Can you work these out from the model? Positions are in its coordinate system, mm. Give positions to 0.01 mm unless a question says otherwise; leave off trailing zeros. Write each loop counter-clockwise with the first axis right and the second up, starting at its lowest first coordinate (ties: lowest second). Pieces come first, ordered by that corner, then holes.
1. Suppose I cut it at B-B (z = -0.4). Please give me the cut outline in (x, y), and give its area (3 significant figures).
2. Suppose I cut it at A-A (x = -38.1). Please give me the cut outline in (y, z).
3. Suppose I cut it at D-D (x = 12.7). Please give me the cut outline in (y, z), and give its area (3 significant figures).
4. Suppose I cut it at C-C (y = 12.7). Please give me the cut outline in (x, z).
5. If I drill on probe 1 along X at (y, z) = (12.7, 1.25); probe 2 along X at (y, z) = (13, 0.7); probe 3 along Y at (x, z) = (12.7, 0.85), over which ranges is the centre line in solid material (lowest first)?
```python
from build123d import *

# Parameters (mm, degrees)
SKETCH1_R           = 3.2639
BOSS_EXTRUDE1_DEPTH = 2.38125


with BuildPart() as part:
    # Sketch1 → Boss-Extrude1 (new, symmetric)
    with BuildSketch(Plane.XY):
        Polygon((76.2, 25.4), (25.4, 76.2), (0, 76.2), (-50.8, 25.4), (-50.8, 0), (0, 0), (76.2, 0), align=None)
        with Locations(Location((12.7, 12.7, 0), (0, 0, 180))):
            Circle(SKETCH1_R, mode=Mode.SUBTRACT)
        with Locations(Location((38.1, 12.7, 0), (0, 0, 180))):
            Circle(SKETCH1_R, mode=Mode.SUBTRACT)
        with Locations(Location((63.5, 12.7, 0), (0, 0, 180))):
            Circle(SKETCH1_R, mode=Mode.SUBTRACT)
        with Locations(Location((12.7, 38.1, 0), (0, 0, 180))):
            Circle(SKETCH1_R, mode=Mode.SUBTRACT)
        with Locations(Location((12.7, 63.5, 0), (0, 0, 180))):
            Circle(SKETCH1_R, mode=Mode.SUBTRACT)
        with Locations(Location((-38.1, 12.7, 0), (0, 0, 180))):
            Circle(SKETCH1_R, mode=Mode.SUBTRACT)
        with Locations(Location((-12.7, 12.7, 0), (0, 0, 180))):
            Circle(SKETCH1_R, mode=Mode.SUBTRACT)
    extrude(amount=BOSS_EXTRUDE1_DEPTH, both=True)


solid = part.part
```
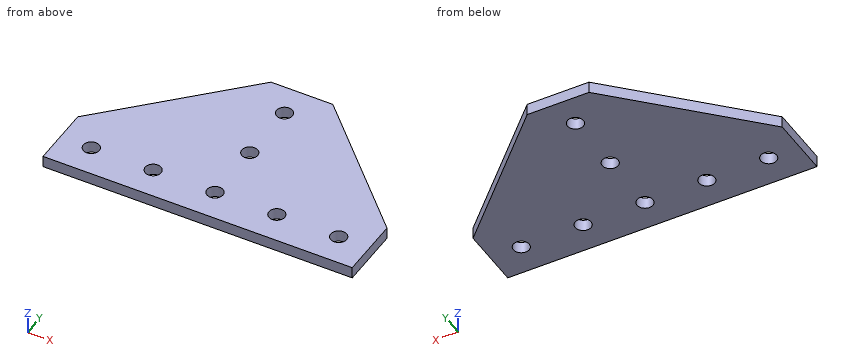
Checks:
1. outline: (-50.8, 0) - (76.2, 0) - (76.2, 25.4) - (25.4, 76.2) - (0, 76.2) - (-50.8, 25.4) - close; hole circle Ø6.53 at (-38.1, 12.7); hole circle Ø6.53 at (-12.7, 12.7); hole circle Ø6.53 at (12.7, 12.7); hole circle Ø6.53 at (12.7, 38.1); hole circle Ø6.53 at (12.7, 63.5); hole circle Ø6.53 at (38.1, 12.7); hole circle Ø6.53 at (63.5, 12.7)
1. area: 6,860 mm2
2. outline: (0, -2.38) - (9.44, -2.38) - (9.44, 2.38) - (0, 2.38) - close; (15.96, -2.38) - (38.1, -2.38) - (38.1, 2.38) - (15.96, 2.38) - close
3. outline: (0, -2.38) - (9.44, -2.38) - (9.44, 2.38) - (0, 2.38) - close; (15.96, -2.38) - (34.84, -2.38) - (34.84, 2.38) - (15.96, 2.38) - close; (41.36, -2.38) - (60.24, -2.38) - (60.24, 2.38) - (41.36, 2.38) - close; (66.76, -2.38) - (76.2, -2.38) - (76.2, 2.38) - (66.76, 2.38) - close
3. area: 270 mm2
4. outline: (-50.8, -2.38) - (-41.36, -2.38) - (-41.36, 2.38) - (-50.8, 2.38) - close; (-34.84, -2.38) - (-15.96, -2.38) - (-15.96, 2.38) - (-34.84, 2.38) - close; (-9.44, -2.38) - (9.44, -2.38) - (9.44, 2.38) - (-9.44, 2.38) - close; (15.96, -2.38) - (34.84, -2.38) - (34.84, 2.38) - (15.96, 2.38) - close; (41.36, -2.38) - (60.24, -2.38) - (60.24, 2.38) - (41.36, 2.38) - close; (66.76, -2.38) - (76.2, -2.38) - (76.2, 2.38) - (66.76, 2.38) - close
5. probe 1: x = -50.8 to -41.36, -34.84 to -15.96, -9.44 to 9.44, 15.96 to 34.84, 41.36 to 60.24, 66.76 to 76.2
5. probe 2: x = -50.8 to -41.35, -34.85 to -15.95, -9.45 to 9.45, 15.95 to 34.85, 41.35 to 60.25, 66.75 to 76.2
5. probe 3: y = 0 to 9.44, 15.96 to 34.84, 41.36 to 60.24, 66.76 to 76.2
